from build123d import *

# Parameters (mm, degrees)
SKETCH_1_R      = 8
EXTRUDE_1_DEPTH = 24
SKETCH_2_R      = 42
SKETCH_2_R_2    = 8
EXTRUDE_2_DEPTH = 18
EXTRUDE_3_DEPTH = 18


with BuildPart() as part:
    # 草图1 → 凸台-拉伸1 (new body)
    with BuildSketch(Plane.XY):
        Circle(SKETCH_1_R)
        with BuildLine():
            Line((4.89403723, 1.434712371), (-4.42388764, 2.537561456))
            ThreePointArc((-4.42388764, 2.537561456), (-0.599440727, -5.06464913), (4.89403723, 1.434712371))
        make_face(mode=Mode.SUBTRACT)
    extrude(amount=EXTRUDE_1_DEPTH)

    # 草图2 → 凸台-拉伸2 (add)
    with BuildSketch(Plane.XY):
        Circle(SKETCH_2_R)
        Circle(SKETCH_2_R_2, mode=Mode.SUBTRACT)
    extrude(amount=EXTRUDE_2_DEPTH)

    # 草图3 → 凸台-拉伸3 (add)
    with BuildSketch(Plane.XY):
        with BuildLine():
            Line((37.532556284, 2.035291149), (41.987004924, 1.044709313))
            ThreePointArc((41.987004924, 1.044709313), (42, 0), (41.987004924, -1.044709313))
            Line((41.987004924, -1.044709313), (37.532556284, -2.035291149))
            ThreePointArc((37.532556284, -2.035291149), (37.5877, 0), (37.532556284, 2.035291149))
        make_face()
    extrude(amount=EXTRUDE_3_DEPTH)


solid = part.part
Geometry: final body of the model. Coordinates: model frame, mm. A direction names the side the tool comes from. Give positions to 0.01 mm unless a question says otherwise; leave off trailing zeros. Write each loop counter-clockwise with the first axis right and the second up, starting at its lowest first coordinate (ties: lowest second). Pieces come first, ordered by that corner, then holes. Notation, with made-up numbers: (0, -15.5) - (48, -15.5) arc R13 ccw to (48, 9.5) - close; hole circle Ø7 at (-13.5, 29). An arc over 180 degrees is marked (long way). Return JSON: item names as keys, results as strings. Group by question number.
1) Mould query, pull axis X, two halves, no side actions, for faces 1 (the flat face through (9, 1, 18)), 2 (the flat face through (0.3, 1.98, 11.83)), 3 (the cylindrical face through (40.06, 12.62, 8.87)). Classes: released by +X, released by -X, zero draft, split by the parting line, or undercut.
2) Section B-B on x = 0. Return the cut outline in (y, z), plus the area to 3 significant figures.
3) Section A-A on y = 0. Return the cut outline in (x, z).
4) Line query: line 1 (X direction, y = 0, z = 16.5); line 2 (Y direction, x = -0.5, z = 3.75); line 3 (Z direction, x = -21.5, y = -35). Output: solid intervals per line, ascending.
5) First-contact query: P1, Ø2, axis at x = -8.5, y = 10.5, coming from the +Z side; P2, Ø4, axis at x = 4, z = 7, coming from the +Y side; P3, Ø2, axis at y = -23.5, z = 13.5, coming from the +X side. Flat tips, straight axial feed; report the tip coordinate or a pass-through.
6) Set-up query: faces 4 (the flat face through (9, 1, 0)), 5 (the cylindrical face through (-1.73, -7.81, 20.96)). Return all of +Z, -Z, +X, -X, +Y, -Y with unobstructed straight access to the full face (end or side cutting, diameter ignored); none if empty.
7) Section D-D on z = 12.25. Return the cut outline in (x, y).
8) Section C-C on z = 19.5. Return the cut outline in (x, y), plus the area to 3 significant figures.
Filled in:
{
 "1": {"face 1": "zero draft", "face 2": "undercut", "face 3": "split by the parting line"},
 "2": {"outline": "(-42, 0) - (-5.1, 0) - (-5.1, 24) - (-8, 24) - (-8, 18) - (-42, 18) - close; (2.01, 0) - (42, 0) - (42, 18) - (8, 18) - (8, 24) - (2.01, 24) - close", "area": "1,440 mm^2"},
 "3": {"outline": "(-42, 0) - (-5.1, 0) - (-5.1, 24) - (-8, 24) - (-8, 18) - (-42, 18) - close; (5.1, 0) - (42, 0) - (42, 18) - (8, 18) - (8, 24) - (5.1, 24) - close"},
 "4": {"line 1": "x = -42 to -5.1, 5.1 to 42", "line 2": "y = -42 to -5.08, 2.07 to 42", "line 3": "z = 0 to 18"},
 "5": {"P1": "stops at z = 18", "P2": "stops at y = 41.95", "P3": "stops at x = 35.46"},
 "6": {"face 4": "-Z, +X, -X, +Y, -Y", "face 5": "+Z"},
 "7": {"outline": "circle Ø84 at (0, 0); hole (-4.42, 2.54) arc R5.1 ccw (long way) to (4.89, 1.43) - close"},
 "8": {"outline": "circle Ø16 at (0, 0); hole (-4.42, 2.54) arc R5.1 ccw (long way) to (4.89, 1.43) - close", "area": "140 mm^2"}
}
